```python
from build123d import *

# Parameters (mm, degrees)
F0_R     = 75.614266
F1_DEPTH = 12.7
F2_R     = 14.018878
F2_R_2   = 15.125501
F3_DEPTH = 12.7
F4_SIZE  = 5.08
F5_SIZE  = 5.08


with BuildPart() as f1:
    # F0 (on Front) → F1 (new body)
    with BuildSketch(Plane.XZ):
        Circle(F0_R)
    extrude(amount=F1_DEPTH)

    # F2 (on face) → F3 (join)
    with BuildSketch(Plane.XZ.offset(12.7)):
        with Locations((28.639855, 15.135232)):
            Circle(F2_R)
        with Locations((-33.897843, 12.963785)):
            Circle(F2_R_2)
    extrude(amount=F3_DEPTH)

    # F4
    f4_edges = [f1.edges().sort_by_distance(p)[0] for p in [
        (-49.023345, -25.4, 12.963785),
        (14.620977, -25.4, 15.135232),
    ]]
    chamfer(f4_edges, length=F4_SIZE)

    # F5
    f5_edges = [f1.edges().sort_by_distance(p)[0] for p in [
        (-75.614266, -12.7, 0),
        (-49.023345, -12.7, 12.963785),
        (14.620977, -12.7, 15.135232),
    ]]
    chamfer(f5_edges, length=F5_SIZE)


solid = f1.part
```
Build history of the part. All positions in model axes, mm. A direction names the side the tool comes from. Give positions to 0.01 mm unless a question says otherwise; leave off trailing zeros. Loops run counter-clockwise (first coordinate to the right, second up) from the corner with the lowest first, then second, coordinate; pieces in that order, holes last.
1) Drop flat-ended pins along their axis: P1, Ø8, axis at y = -14.5, z = 34.5, coming from the +X side; P2, Ø12, axis at y = -3.5, z = -60, coming from the +X side; P3, Ø6, axis at x = -53.5, y = -5.5, coming from the -Z side; P4, Ø12, axis at y = -21, z = 53.5, coming from the +X side. Give the stop position or say it passes through.
Values follow:
P1: stops at x = 64.49
P2: stops at x = 52.93
P3: stops at z = -56.28
P4: passes through
2) Band-saw the part on C-C on y = -5. List the corners of the cut face in (x, z), then the cut area to 3 significant figures.
Values follow:
outline: circle Ø151.23 at (0, 0)
area: 18,000 mm2
3) Probe line 1 along Y through (x, z) = (10.5, -65.5); line 2 along Z through (x, y) = (0, -2); line 3 along X through (y, z) = (-21.5, 18). List the from-to ranges inside material, lowest first.
Values follow:
line 1: y = -12.7 to 0
line 2: z = -75.61 to 75.61
line 3: x = -46.9 to -20.89, 16.12 to 41.16
4) Band-saw the part on B-B on y = -15.5. List the corners of the cut face in (x, z).
Values follow:
outline: circle Ø34.81 at (-33.9, 12.96); circle Ø32.6 at (28.64, 15.14)
5) Two-plate mould, pull along X, no slides. Class faces 3 (the face through (-1, 0, 1)), 4 (the face through (-60.005, -3.757, -46.01)), 5 (the face through (18.3, -19, 24.6)): released by +X, released by -X, zero draft, split by the parting line, or undercut.
Values follow:
face 3: zero draft
face 4: split by the parting line
face 5: undercut
6) 3-axis set-ups, long thin cutter, end or side, ignore diameter. For faces 1 (the face through (-1, -12.7, 1)), 2 (the face through (29, -25.4, 15)): which of +Z, -Z, +X, -X, +Y, -Y reach the whole face in a straight line?
Values follow:
face 1: -Y
face 2: +Z, -Z, +X, -X, -Y
7) Band-saw the part on A-A on x = 0. List the corners of the cut face in (y, z), then the cut area to 3 significant figures.
Values follow:
outline: (-12.7, -70.53) - (-7.62, -75.61) - (0, -75.61) - (0, 75.61) - (-7.62, 75.61) - (-12.7, 70.53) - close
area: 1,890 mm2
